from build123d import *

# Parameters (mm, degrees)
SKETCH1_W           = 43
SKETCH1_H           = 17.8
BOSS_EXTRUDE1_DEPTH = 3
SKETCH2_W           = 22
SKETCH2_H           = 2.9
CUT_EXTRUDE1_DEPTH  = 4
SKETCH3_W           = 22
SKETCH3_H           = 2.9
CUT_EXTRUDE2_DEPTH  = 4
CUT_EXTRUDE3_DEPTH  = 2
CUT_EXTRUDE4_DEPTH  = 4
SKETCH6_W           = 10
SKETCH6_H           = 2
CUT_EXTRUDE5_DEPTH  = 15
CHAMFER1_SIZE       = 0.4


with BuildPart() as part:
    # Sketch1 → Boss-Extrude1 (new body)
    with BuildSketch(Plane(origin=(0, 38, 0), x_dir=(1, 0, 0), z_dir=(0, 1, 0))):
        with Locations((-6.5, 6)):
            Rectangle(SKETCH1_W, SKETCH1_H)
    extrude(amount=-BOSS_EXTRUDE1_DEPTH)

    # Sketch2 → Cut-Extrude1 (cut, through all)
    with BuildSketch(Plane.XZ.offset(-35)):
        with Locations((4, 1.45)):
            Rectangle(SKETCH2_W, SKETCH2_H)
    extrude(amount=-CUT_EXTRUDE1_DEPTH, mode=Mode.SUBTRACT)

    # Sketch3 → Cut-Extrude2 (cut, through all)
    with BuildSketch(Plane.XZ.offset(-35)):
        with Locations((4, -13.45)):
            Rectangle(SKETCH3_W, SKETCH3_H)
    extrude(amount=-CUT_EXTRUDE2_DEPTH, mode=Mode.SUBTRACT)

    # Sketch4 → Cut-Extrude3 (cut)
    with BuildSketch(Plane(origin=(0, 38, 0), x_dir=(-1, 0, 0), z_dir=(0, 1, 0))):
        with BuildLine():
            Line((22.9, -11.9), (22.9, -3.4))
            ThreePointArc((22.9, -3.4), (20.9, -1.4), (18.9, -3.4))
            Line((18.9, -3.4), (18.9, -11.9))
            ThreePointArc((18.9, -11.9), (20.9, -13.9), (22.9, -11.9))
        make_face()
    extrude(amount=-CUT_EXTRUDE3_DEPTH, mode=Mode.SUBTRACT)

    # Sketch5 → Cut-Extrude4 (cut, through all)
    with BuildSketch(Plane.XZ.offset(-35)):
        with BuildLine():
            Line((-22.1, -3.4), (-22.1, -11.9))
            ThreePointArc((-22.1, -11.9), (-20.9, -13.1), (-19.7, -11.9))
            Line((-19.7, -11.9), (-19.7, -3.4))
            ThreePointArc((-19.7, -3.4), (-20.9, -2.2), (-22.1, -3.4))
        make_face()
    extrude(amount=-CUT_EXTRUDE4_DEPTH, mode=Mode.SUBTRACT)

    # Sketch6 → Cut-Extrude5 (cut)
    with BuildSketch(Plane(origin=(15, 0, 0), x_dir=(0, 0, -1), z_dir=(1, 0, 0))):
        with Locations((6, 37)):
            Rectangle(SKETCH6_W, SKETCH6_H)
    extrude(amount=-CUT_EXTRUDE5_DEPTH, mode=Mode.SUBTRACT)

    # Chamfer1
    chamfer1_edges = [part.edges().sort_by_distance(p)[0] for p in [
        (15, 38, -0.5),
        (15, 35, -6),
        (-7, 36.5, 2.9),
        (4, 38, 0),
        (15, 36.5, 0),
        (-7, 38, 1.45),
        (-7, 35, 1.45),
        (4, 35, 0),
        (-17.5, 38, -14.9),
        (-17.5, 35, -14.9),
        (15, 36.5, -12),
        (-7, 38, -13.45),
        (-7, 36.5, -14.9),
        (4, 38, -12),
        (4, 35, -12),
        (-7, 35, -13.45),
        (-20.9, 38, -13.9),
        (-22.9, 38, -7.65),
        (-20.9, 38, -1.4),
        (-28, 35, -6),
        (-18.9, 38, -7.65),
        (-17.5, 38, 2.9),
        (-28, 38, -6),
        (-20.9, 35, -2.2),
        (-22.1, 35, -7.65),
        (-20.9, 35, -13.1),
        (-19.7, 35, -7.65),
        (-28, 36.5, -14.9),
        (15, 38, -11.5),
        (-28, 36.5, 2.9),
        (-17.5, 35, 2.9),
    ]]
    chamfer(chamfer1_edges, length=CHAMFER1_SIZE)


solid = part.part
Model file for the job. Use its own axes, mm. A direction names the side the tool comes from. Give positions to 0.01 mm unless a question says otherwise; leave off trailing zeros. Write each loop counter-clockwise with the first axis right and the second up, starting at its lowest first coordinate (ties: lowest second). Pieces come first, ordered by that corner, then holes. Notation, with made-up numbers: M 39.25,81.25 L 61.25,81.25 A22 ccw 61.25,106.25 Z; hole C 5,64.5 d11. An arc over 180 degrees is marked long. One line per item, written item: value. Start each with the question number.
Q1. Probe probe 1 along X at (y, z) = (36.2, -8); probe 2 along X at (y, z) = (35.7, -5.25); probe 3 along Z at (x, y) = (-2, 35.8). List the from-to ranges inside material, lowest first. Write a range as [from, to].
Q2. Saw through at C-C, the plane y = 36.85. Write the cut outline in (x, z).
Q3. Saw through at B-B, the plane z = -9. Write the cut outline in (x, y).
Q4. Saw through at A-A, the plane x = -20.9. Write the cut outline in (y, z), plus the area to 3 significant figures.
Q5. Two-plate mould, pull along Z, no slides. Class faces 1 (the cylindrical face through (-20.9, 35.7, -2.2)), 2 (the flat face through (4, 36, 0)), 3 (the flat face through (15, 35.8, -5.6)): +Z half, -Z half, draft (parallel to the pull), parting line (faces both ways), or undercut.
Q6. 3-axis set-ups, long thin cutter, end or side, ignore diameter. For faces 4 (the cylindrical face through (-20.9, 35.7, -13.1)), 5 (the conical face through (-20.93, 35.29, -13.21)), 6 (the flat face through (-18.9, 37, -8)), 7 (the flat face through (8, 36, -6)), 8 (the flat face through (4, 36, -12)): which of +Z, -Z, +X, -X, +Y, -Y reach the whole face in a straight line?
Q7. Drop flat-ended pins along their axis: pin 1 Ø0.7 at (y, z) = (37, 1.5) entering from +X; pin 2 Ø3 at (x, z) = (10.5, -3.5) entering from +Y; pin 3 Ø1.5 at (x, y) = (0, 36.5) entering from +Z. Give the stop position or say it passes through.
Q8. Saw through at D-D, the plane x = -2. Write the cut outline in (y, z), plus the area to 3 significant figures.
Output values:
1. probe 1: x = [-28, -22.9], [-18.9, 0]
1. probe 2: x = [-28, -22.1], [-19.7, 15]
1. probe 3: z = [-12, 0]
2. outline: M -28,-14.5 L -27.6,-14.9 L -7.4,-14.9 L -7,-14.5 L -7,-12 L 14.6,-12 L 15,-11.6 L 15,-11 L 0,-11 L 0,-1 L 15,-1 L 15,-0.4 L 14.6,0 L -7,0 L -7,2.5 L -7.4,2.9 L -27.6,2.9 L -28,2.5 Z; hole M -22.9,-11.9 A2 ccw -18.9,-11.9 L -18.9,-3.4 A2 ccw -22.9,-3.4 Z
3. outline: M -28,35.4 L -27.6,35 L -22.5,35 L -22.1,35.4 L -22.1,36 L -22.9,36 L -22.9,37.6 L -23.3,38 L -27.6,38 L -28,37.6 Z; M -19.7,35.4 L -19.3,35 L 14.6,35 L 15,35.4 L 15,36 L 0,36 L 0,38 L -18.5,38 L -18.9,37.6 L -18.9,36 L -19.7,36 Z
4. outline: M 35,-14.5 L 35.4,-14.9 L 37.6,-14.9 L 38,-14.5 L 38,-14.3 L 37.6,-13.9 L 36,-13.9 L 36,-13.1 L 35.4,-13.1 L 35,-13.5 Z; M 35,-1.8 L 35.4,-2.2 L 36,-2.2 L 36,-1.4 L 37.6,-1.4 L 38,-1 L 38,2.5 L 37.6,2.9 L 35.4,2.9 L 35,2.5 Z
4. area: 16.9 mm²
5. face 1: undercut
5. face 2: +Z half
5. face 3: draft
6. face 4: +Y, -Y
6. face 5: -Y
6. face 6: +Y
6. face 7: +X, +Y
6. face 8: -Z, +X, +Y, -Y
7. pin 1: stops at x = -7
7. pin 2: stops at y = 36
7. pin 3: stops at z = 0
8. outline: M 35,-11.6 L 35.4,-12 L 37.6,-12 L 38,-11.6 L 38,-0.4 L 37.6,0 L 35.4,0 L 35,-0.4 Z
8. area: 35.7 mm²
